For this review, use the dimensioned drawing (mm, ordinates from the lowest corner) and the shaded views. Give positions to 0.01 mm unless a question says otherwise; leave off trailing zeros. Loops run counter-clockwise (first coordinate to the right, second up) from the corner with the lowest first, then second, coordinate; pieces in that order, holes last. Notation, with made-up numbers: (5.5, 35) - (51.5, 35) arc R38 cw to (51.5, 74) - close; hole circle Ø7 at (61.5, 6). An arc over 180 degrees is marked (long way). Put each result on its own line as item: value.
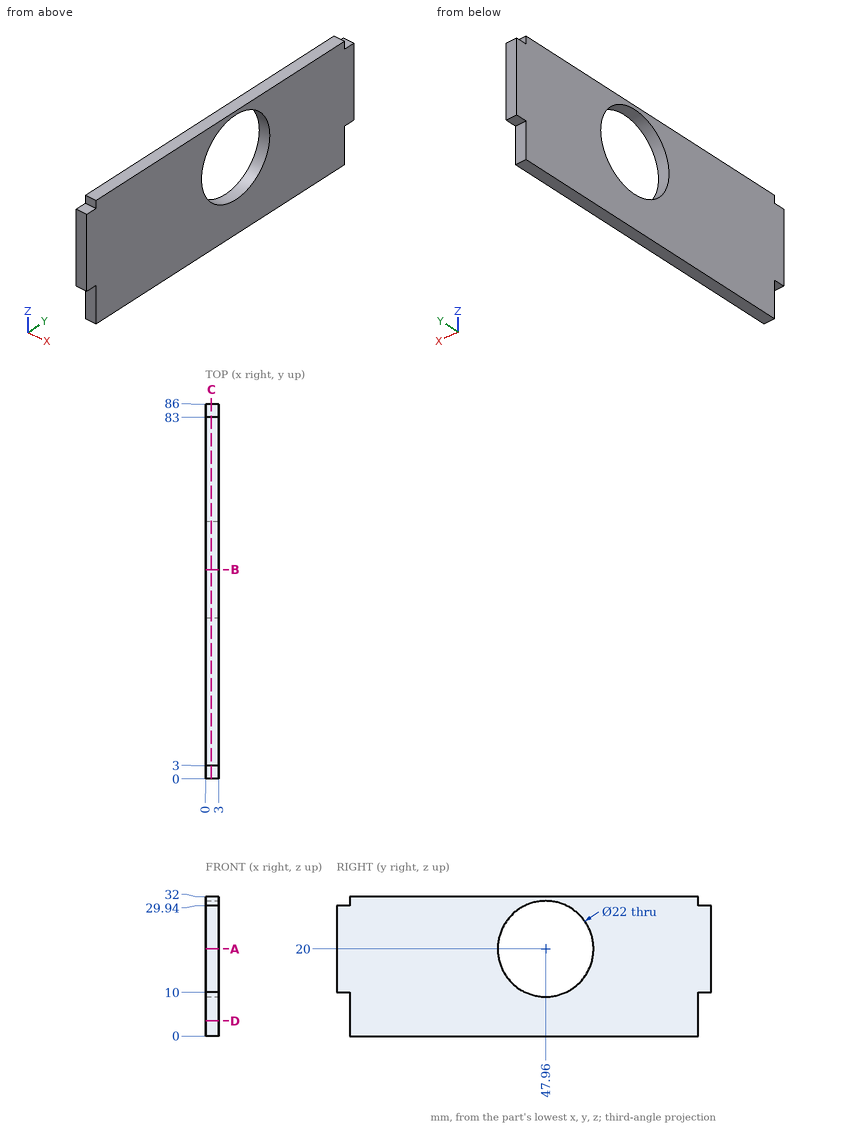
1) Take a section at D-D on z = 3.5. State the section outline as (x, y) points, and give its area (3 significant figures).
Geometry check:
outline: (0, 3) - (3, 3) - (3, 83) - (0, 83) - close
area: 240 mm²
2) Insertion check: pin 1 Ø1 at (x, z) = (2, 5.5) entering from +Y; pin 2 Ø1.5 at (x, z) = (2, 5) entering from -Y; pin 3 Ø1.5 at (x, y) = (2, 85) entering from +Z. Each pin has a flat end and moves straight along its axis. Give the tip position at first contact, or say it passes through.
Geometry check:
pin 1: stops at y = 83
pin 2: stops at y = 3
pin 3: stops at z = 29.94
3) Take a section at C-C on x = 1.3. State the section outline as (y, z) points, and give its area (3 significant figures).
Geometry check:
outline: (0, 10) - (3, 10) - (3, 0) - (83, 0) - (83, 10) - (86, 10) - (86, 29.94) - (83, 29.94) - (83, 32) - (3, 32) - (3, 29.94) - (0, 29.94) - close; hole circle Ø22 at (47.96, 20)
area: 2,300 mm²
4) Wall thickness on line 1 (Z direction, x = 1.4, y = 47.96); line 2 (Y direction, x = 0.2, z = 5.5); line 3 (Y direction, x = 1.35, z = 22.5): over which ranges is each line inside the solid? List them lowest first.
Geometry check:
line 1: z = 0 to 9, 31 to 32
line 2: y = 3 to 83
line 3: y = 0 to 37.25, 58.67 to 86
5) Take a section at A-A on z = 20. State the section outline as (x, y) points.
Geometry check:
outline: (0, 0) - (3, 0) - (3, 36.96) - (0, 36.96) - close; (0, 58.96) - (3, 58.96) - (3, 86) - (0, 86) - close
6) Take a section at B-B on y = 47.96. State the section outline as (x, z) points, and give its area (3 significant figures).
Geometry check:
outline: (0, 0) - (3, 0) - (3, 9) - (0, 9) - close; (0, 31) - (3, 31) - (3, 32) - (0, 32) - close
area: 30.0 mm²
